Can you work these out from the model? Positions are in its coordinate system, mm. Face numbers are marked on the shaded views. A direction names the side the tool comes from. Give positions to 0.01 mm unless a question says otherwise; leave off trailing zeros. Order: outer loops, then holes, each group sorted by start corner. A loop starts at its lowest first (then second) coordinate and runs counter-clockwise, first axis right, second up. Notation, with made-up numbers: (64.25, -35.5) - (69.25, -35.5) arc R30 ccw to (69.25, -4.5) - close; hole circle Ø7 at (-24, 9.5). An arc over 180 degrees is marked (long way). Answer as a JSON object with one key per item and string values.
```python
from build123d import *

# Parameters (mm, degrees)
F0_W     = 106
F0_H     = 64
F0_R     = 20
F1_DEPTH = 40
F3_DEPTH = 120
F4_R     = 1.5
F5_T     = -3


with BuildPart() as f1:
    # F0 (on Front) → F1 (new body)
    with BuildSketch(Plane.XZ):
        with Locations((0.0056690624, 0.0035208468)):
            Rectangle(F0_W, F0_H)
        with Locations((0.0056690624, 0.0035208468)):
            Circle(F0_R, mode=Mode.SUBTRACT)
    extrude(amount=F1_DEPTH)

    # F2 (on face) → F3 (cut)
    with BuildSketch(Plane.YZ.offset(53.0056690624)):
        Polygon((-40, 32.0035208468), (-40, -31.9964791532), (-10, 32.0035208468), align=None)
    extrude(amount=-F3_DEPTH, mode=Mode.SUBTRACT)

    # F4
    f4_edges = [f1.edges().sort_by_distance(p)[0] for p in [
        (53.005669, -5, 32.003521),
        (-52.994331, -5, 32.003521),
        (-52.994331, -20, -31.996479),
        (53.005669, -20, -31.996479),
    ]]
    fillet(f4_edges, radius=F4_R)

    # F5
    f5_openings = [f1.faces().sort_by_distance(p)[0] for p in [
        (0.005669, -39.459251, -30.84288),
        (-19.994331, -17.1875, 0.003521),
    ]]
    offset(amount=F5_T, openings=f5_openings)


solid = f1.part
```
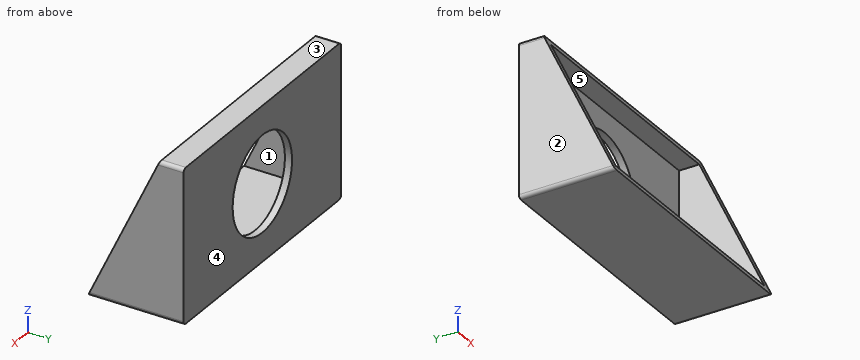
Q1. We'd pull the mould along X, two halves only. Please class the marked faces 1, 2 and 3: released by +X, released by -X, zero draft, split by the parting line, or undercut.
Recorded:
{"face 1": "undercut", "face 2": "released by -X", "face 3": "zero draft"}
Q2. I'm going to push flat-ended pins straight in: pin 1 Ø1 at (x, z) = (29, 14) entering from +Y; pin 2 Ø4 at (x, y) = (16.5, -24.5) entering from +Z; pin 3 Ø6 at (x, z) = (-36.5, -5.5) entering from -Y. Where does each tip first touch, or does it pass through?
Recorded:
{"pin 1": "stops at y = 0", "pin 2": "stops at z = -29", "pin 3": "stops at y = -3"}
Q3. I need wall thicknesses on L1, parallel to Z at x = 33, y = -9.5; L2, parallel to X at y = -22, z = -20; L3, parallel to Y at x = -30.5, z = 10. Which ranges of each line are inside material? Lowest first, please.
Recorded:
{"L1": "z = -32 to -29, 29 to 32", "L2": "x = -52.99 to -49.99, 50.01 to 53.01", "L3": "y = -3 to 0"}
Q4. If we section it at B-B, the plane x = 12.5: Please give me the cut outline in (y, z).
Recorded:
{"outline": "(-40, -32) - (0, -32) - (0, -15.61) - (-3, -15.61) - (-3, -29) - (-38.59, -29) - close; (-11.41, 29) - (-3, 29) - (-3, 15.62) - (0, 15.62) - (0, 32) - (-10, 32) - close"}
Q5. If we section it at A-A, the plane z = 2: Please give me the cut outline in (x, y), then the cut area to 3 significant figures.
Recorded:
{"outline": "(-52.99, -24.06) - (-49.99, -24.06) - (-49.99, -3) - (-19.89, -3) - (-19.89, 0) - (-52.99, 0) - close; (19.91, -3) - (50.01, -3) - (50.01, -24.06) - (53.01, -24.06) - (53.01, 0) - (19.91, 0) - close", "area": "325 mm^2"}
Q6. Which directions (+Z, -Z, +X, -X, +Y, -Y) give clear straight access to the entire face, cutting with the end or side of a thin tool? Please do the marked faces 4 and 5.
Recorded:
{"face 4": "+Z, -Z, +X, -X, +Y", "face 5": "-Y"}
Q7. If we section it at C-C, the plane y = -7.5: Please give me the cut outline in (x, z), then the cut area to 3 significant figures.
Recorded:
{"outline": "(-52.99, -30.5) arc R1.5 ccw to (-51.49, -32) - (51.51, -32) arc R1.5 ccw to (53.01, -30.5) - (53.01, 30.5) arc R1.5 ccw to (51.51, 32) - (-51.49, 32) arc R1.5 ccw to (-52.99, 30.5) - close; hole (-49.99, -29) - (50.01, -29) - (50.01, 29) - (-49.99, 29) - close", "area": "982 mm^2"}
Q8. If we section it at D-D, the plane x = -36: Please give me the cut outline in (y, z), then the cut area to 3 significant figures.
Recorded:
{"outline": "(-40, -32) - (0, -32) - (0, 32) - (-10, 32) - (-11.41, 29) - (-3, 29) - (-3, -29) - (-38.59, -29) - close", "area": "324 mm^2"}
